Can you work these out from the model? Positions are in its coordinate system, mm. A direction names the side the tool comes from. Round coordinates to 2 decimals unless told otherwise and drop trailing zeros. Write each loop counter-clockwise with the first axis right and the second up, starting at its lowest first coordinate (ties: lowest second). Pieces come first, ordered by that corner, then holes. Notation, with made-up numbers: M 57,26.25 L 115,26.25 A7 ccw 115,37.25 Z; hole C 46,68.25 d11. An arc over 180 degrees is marked long. Answer in a Markdown table with one row per item. Add a question column.
(1) Suppose I cut it at A-A, the plane z = 54.5. Write out the boundary of the cut face in (x, y).
(2) Suppose I cut it at C-C, the plane y = 3.75. Write out the boundary of the cut face in (x, z), then the cut area to 3 significant figures.
(3) Suppose I cut it at B-B, the plane x = 0. Write out the boundary of the cut face in (y, z).
(4) I'm going to push flat-ended pins straight in: pin 1 (6 mm diameter, centred on y = -4.5, z = 14, fed in from +X); pin 2 (5 mm diameter, centred on y = 3.5, z = 15, fed in from +X) (3 decimals); pin 3 (2 mm diameter, centred on x = 5, y = -3.5, fed in from +Z). Where does each tip first touch, or does it pass through?
(5) If I drill on probe 1 along Z at (x, y) = (-3.5, -0.75); probe 2 along X at (y, z) = (3.75, 85); probe 3 along X at (y, z) = (-0.5, 94), over which ranges is the centre line in solid material (lowest first)?
(6) For faces 1 (the face through (0, 3, 88.9)), 2 (the face through (0, 1.658, 99)), 3 (the face through (0, 6.35, -8)), which set-ups out of +Z, -Z, +X, -X, +Y, -Y let a thin tool reach every point of the face, with its end or its side?
from build123d import *

# Parameters (mm, degrees)
BOSS_EXTRUDE1_DEPTH = 107.95
CUT_EXTRUDE1_DEPTH  = 19.05


with BuildPart() as part:
    # Sketch1 → Boss-Extrude1 (new, symmetric)
    with BuildSketch(Plane.XY):
        Polygon((3.666174209, 6.35), (-3.666174209, 6.35), (-7.332348419, 0), (-3.666174209, -6.35), (3.666174209, -6.35), (7.332348419, 0), align=None)
    extrude(amount=BOSS_EXTRUDE1_DEPTH, both=True)

    # Sketch2 → Cut-Extrude1 (cut)
    with BuildSketch(Plane.XY.offset(107.95)):
        Polygon((-3.666174209, 6.35), (-7.332348419, 0), (-3.666174209, -6.35), (3.666174209, -6.35), (7.332348419, 0), (3.666174209, 6.35), align=None)
        with BuildLine():
            Line((-2.5, 1.658312395), (2.5, 1.658312395))
            ThreePointArc((2.5, 1.658312395), (0, -3), (-2.5, 1.658312395))
        make_face(mode=Mode.SUBTRACT)
    extrude(amount=-CUT_EXTRUDE1_DEPTH, mode=Mode.SUBTRACT)


solid = part.part
Calculated:
| question | item | result |
|---|---|---|
| 1 | outline | M -7.33,0 L -3.67,-6.35 L 3.67,-6.35 L 7.33,0 L 3.67,6.35 L -3.67,6.35 Z |
| 2 | outline | M -5.17,-107.95 L 5.17,-107.95 L 5.17,88.9 L -5.17,88.9 Z |
| 2 | area | 2,030 mm² |
| 3 | outline | M -6.35,-107.95 L 6.35,-107.95 L 6.35,88.9 L 1.66,88.9 L 1.66,107.95 L -3,107.95 L -3,88.9 L -6.35,88.9 Z |
| 4 | pin 1 | x = 6.47 |
| 4 | pin 2 | x = 6.755 |
| 4 | pin 3 | z = 88.9 |
| 5 | probe 1 | -107.95 to 88.9 |
| 5 | probe 2 | -5.17 to 5.17 |
| 5 | probe 3 | -2.96 to 2.96 |
| 6 | face 1 | +Z |
| 6 | face 2 | +Z, +X, -X, +Y |
| 6 | face 3 | +Z, -Z, +X, -X, +Y |
